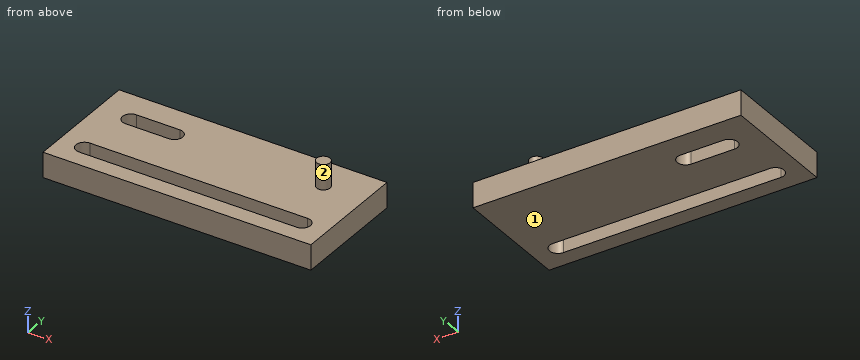
from build123d import *

# Parameters (mm, degrees)
F0_W     = 160
F0_H     = 70
F0_R     = 4
F1_DEPTH = 15
F2_DEPTH = 30


with BuildPart() as f1:
    # F0 (on Top) → F1 (new body)
    with BuildSketch(Plane.XY):
        with Locations((80, 35)):
            Rectangle(F0_W, F0_H)
        with BuildLine():
            ThreePointArc((15, 10), (10, 15), (15, 20))
            Line((15, 20), (145, 20))
            ThreePointArc((145, 20), (150, 15), (145, 10))
            Line((145, 10), (15, 10))
        make_face(mode=Mode.SUBTRACT)
        with BuildLine():
            ThreePointArc((20, 45), (15, 50), (20, 55))
            Line((20, 55), (46, 55))
            ThreePointArc((46, 55), (51, 50), (46, 45))
            Line((46, 45), (20, 45))
        make_face(mode=Mode.SUBTRACT)
        with Locations((135, 50)):
            Circle(F0_R, mode=Mode.SUBTRACT)
        with Locations((135, 50)):
            Circle(F0_R)
    extrude(amount=F1_DEPTH)

    # F0 (on Top) → F2 (join)
    with BuildSketch(Plane.XY):
        with Locations((135, 50)):
            Circle(F0_R)
    extrude(amount=F2_DEPTH)


solid = f1.part
Source: CAD feature listing. Evaluate the final solid. Frame: model axes, mm. Face numbers are marked on the shaded views. A direction names the side the tool comes from. Round coordinates to 2 decimals unless told otherwise and drop trailing zeros. Loops run counter-clockwise (first coordinate to the right, second up) from the corner with the lowest first, then second, coordinate; pieces in that order, holes last.
Q1. Ray query, line 1 (Y direction, x = 36.5, z = 3.5); line 2 (Y direction, x = 83, z = 5); line 3 (Z direction, x = 31, y = 55.5). Return the intervals inside material, ascending.
Q2. First-contact query: P1, Ø1, axis at y = 49, z = 24.5, coming from the +X side; P2, Ø1, axis at y = 21, z = 16, coming from the +X side; P3, Ø2, axis at x = 94.5, y = 57, coming from the +Z side; P4, Ø10, axis at x = 138.5, z = 21, coming from the +Y side. Flat tips, straight axial feed; report the tip coordinate or a pass-through.
Q3. Section C-C, the plane z = 6.75. Return loops of the section in (x, y), plus the area to 3 significant figures.
Q4. Section D-D, the plane x = 41. Return loops of the section in (y, z).
Q5. Section A-A, the plane x = 135. Return loops of the section in (y, z), plus the area to 3 significant figures.
Q6. Access query for the marked faces 1 and 2. Directions: +Z, -Z, +X, -X, +Y, -Y. A direction counts if a zero-diameter tool reaches every point of the face in a straight line with its end or side. Return the directions, or none.
Q7. Section B-B, the plane y = 50. Return loops of the section in (x, z).
Solutions:
1. line 1: y = 0 to 10, 20 to 45, 55 to 70
1. line 2: y = 0 to 10, 20 to 70
1. line 3: z = 0 to 15
2. P1: stops at x = 138.97
2. P2: passes through
2. P3: stops at z = 15
2. P4: stops at y = 54
3. outline: (0, 0) - (160, 0) - (160, 70) - (0, 70) - close; hole (15, 10) - (145, 10) arc R5 ccw to (145, 20) - (15, 20) arc R5 ccw to start; hole (20, 45) - (46, 45) arc R5 ccw to (46, 55) - (20, 55) arc R5 ccw to start
3. area: 9,480 mm2
4. outline: (0, 0) - (10, 0) - (10, 15) - (0, 15) - close; (20, 0) - (45, 0) - (45, 15) - (20, 15) - close; (55, 0) - (70, 0) - (70, 15) - (55, 15) - close
5. outline: (0, 0) - (10, 0) - (10, 15) - (0, 15) - close; (20, 0) - (70, 0) - (70, 15) - (54, 15) - (54, 30) - (46, 30) - (46, 15) - (20, 15) - close
5. area: 1,020 mm2
6. face 1: -Z, +X, -X, +Y, -Y
6. face 2: +Z
7. outline: (0, 0) - (15, 0) - (15, 15) - (0, 15) - close; (51, 0) - (160, 0) - (160, 15) - (139, 15) - (139, 30) - (131, 30) - (131, 15) - (51, 15) - close
